from build123d import *

# Parameters (mm, degrees)
SKETCH1_W           = 120
SKETCH1_H           = 100
BOSS_EXTRUDE1_DEPTH = 20
SKETCH6_W           = 110
SKETCH6_H           = 40
CUT_EXTRUDE1_DEPTH  = 20
SKETCH6_3_W         = 5
SKETCH6_3_H         = 40
BOSS_EXTRUDE4_DEPTH = 20
SKETCH14_W          = 5
SKETCH14_H          = 5
CUT_EXTRUDE2_DEPTH  = 10
SKETCH15_W          = 10
SKETCH15_H          = 10
CUT_EXTRUDE3_DEPTH  = 10
SKETCH16_W          = 3
SKETCH16_H          = 3
SKETCH16_W_2        = 6
SKETCH16_H_2        = 6
CUT_EXTRUDE4_DEPTH  = 5


with BuildPart() as part:
    # Sketch1 → Boss-Extrude1 (new body)
    with BuildSketch(Plane(origin=(0, 0, 0), x_dir=(1, 0, 0), z_dir=(0, 1, 0))):
        Rectangle(SKETCH1_W, SKETCH1_H)
    extrude(amount=BOSS_EXTRUDE1_DEPTH)

    # Sketch6 → Cut-Extrude1 (cut)
    with BuildSketch(Plane.XZ):
        with Locations((0, 25)):
            Rectangle(SKETCH6_W, SKETCH6_H)
    extrude(amount=-CUT_EXTRUDE1_DEPTH, mode=Mode.SUBTRACT)

    # Sketch6_3 → Boss-Extrude4 (add)
    with BuildSketch(Plane.XZ):
        with Locations((-52.5, 25)):
            Rectangle(SKETCH6_3_W, SKETCH6_3_H)
        with Locations((52.5, 25)):
            Rectangle(SKETCH6_3_W, SKETCH6_3_H)
    extrude(amount=-BOSS_EXTRUDE4_DEPTH)

    # Sketch14 → Cut-Extrude2 (cut)
    with BuildSketch(Plane(origin=(0, 20, 0), x_dir=(1, 0, 0), z_dir=(0, 1, 0))):
        with Locations((-57.5, -7.820888862)):
            Rectangle(SKETCH14_W, SKETCH14_H)
        Polygon((-50, -0.320888862), (-60, -0.320888862), (-60, -5.320888862), (-55, -5.320888862), (-55, -10.320888862), (-50, -10.320888862), (-50, -5), align=None)
        Polygon((60, -5.320888862), (60, -0.320888862), (50, -0.320888862), (50, -5), (50, -10.320888862), (55, -10.320888862), (55, -5.320888862), align=None)
        with Locations((57.5, -7.820888862)):
            Rectangle(SKETCH14_W, SKETCH14_H)
    extrude(amount=-CUT_EXTRUDE2_DEPTH, mode=Mode.SUBTRACT)

    # Sketch15 → Cut-Extrude3 (cut)
    with BuildSketch(Plane(origin=(0, 20, 0), x_dir=(1, 0, 0), z_dir=(0, 1, 0))):
        with Locations((-55, 45)):
            Rectangle(SKETCH15_W, SKETCH15_H)
        with Locations((55, 45)):
            Rectangle(SKETCH15_W, SKETCH15_H)
        with Locations((55, -45)):
            Rectangle(SKETCH15_W, SKETCH15_H)
        with Locations((-55, -45)):
            Rectangle(SKETCH15_W, SKETCH15_H)
    extrude(amount=-CUT_EXTRUDE3_DEPTH, mode=Mode.SUBTRACT)

    # Sketch16 → Cut-Extrude4 (cut)
    with BuildSketch(Plane.XZ):
        with Locations((-57.5, 47.5)):
            Rectangle(SKETCH16_W, SKETCH16_H)
        with Locations((57.5, 47.5)):
            Rectangle(SKETCH16_W, SKETCH16_H)
        with Locations((-57.5, 2.5)):
            Rectangle(SKETCH16_W, SKETCH16_H)
        with Locations((57.5, 2.5)):
            Rectangle(SKETCH16_W, SKETCH16_H)
        with Locations((55, -25)):
            Rectangle(SKETCH16_W_2, SKETCH16_H_2)
        with Locations((-55, -25)):
            Rectangle(SKETCH16_W_2, SKETCH16_H_2)
    extrude(amount=-CUT_EXTRUDE4_DEPTH, mode=Mode.SUBTRACT)


solid = part.part
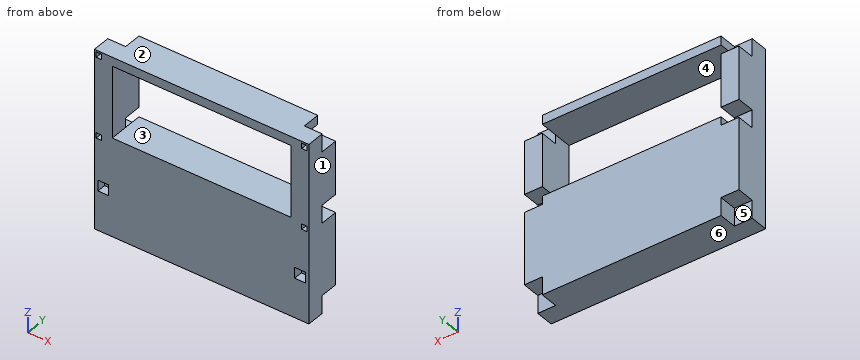
Geometry: final body of the model. Coordinates: model frame, mm. Face numbers are marked on the shaded views. A direction names the side the tool comes from. Round coordinates to 2 decimals unless told otherwise and drop trailing zeros. Write each loop counter-clockwise with the first axis right and the second up, starting at its lowest first coordinate (ties: lowest second). Pieces come first, ordered by that corner, then holes. Notation, with made-up numbers: M -6,63.25 L 44,63.25 A26 ccw 44,101.25 Z; hole C 85,-20 d5. An arc over 180 degrees is marked long. Write item = value, one per line.
Item 1: Section query C-C on y = 8.25. Return loops of the section in (x, z), then the cut area to 3 significant figures.
Findings:
outline = M -60,-50 L 60,-50 L 60,50 L -60,50 Z; hole M -50,5 L 50,5 L 50,45 L -50,45 Z
area = 8,000 mm^2
Item 2: Access query for the marked faces 4, 5 and 6. Directions: +Z, -Z, +X, -X, +Y, -Y. A direction counts if a zero-diameter tool reaches every point of the face in a straight line with its end or side. Return the directions, or none.
Findings:
face_4 = +Y, -Y
face_5 = -Z, -X, +Y
face_6 = -Z, +X, -X, +Y, -Y
Item 3: Section query A-A on x = 0.5. Return loops of the section in (y, z).
Findings:
outline = M 0,-50 L 20,-50 L 20,5 L 0,5 Z; M 0,45 L 20,45 L 20,50 L 0,50 Z
Item 4: Material intervals for line 1 along Z through (x, y) = (-12, 17.25); line 2 along Z through (x, y) = (50.5, 18); line 3 along X through (y, z) = (8, 15), sorted ascending. Write a range as [from, to].
Findings:
line_1 = [-50, 5], [45, 50]
line_2 = [-40, 0.32], [10.32, 40]
line_3 = [-60, -50], [50, 60]
Item 5: Pull-direction query (X, two-part tool) for the marked faces 1, 2 and 3; classes: pulls with the +X half, pulls with the -X half, needs draft (parallel to the pull), parting line crosses it, or undercut.
Findings:
face_1 = pulls with the +X half
face_2 = needs draft
face_3 = undercut
Item 6: Section query D-D on z = -26.5. Return loops of the section in (x, y).
Findings:
outline = M -60,0 L -58,0 L -58,5 L -52,5 L -52,0 L 52,0 L 52,5 L 58,5 L 58,0 L 60,0 L 60,20 L -60,20 Z
Item 7: Pin query (flat end, axial travel): P1, Ø3, axis at x = -55.5, z = -25, coming from the -Y side; P2, Ø5, axis at x = -56, y = 16, coming from the +Z side; P3, Ø5, axis at x = -57, y = 15, coming from the -Z side. Return the tip coordinate at first contact, or that it passes through.
Findings:
P1 = 5
P2 = 40
P3 = -40
Item 8: Section query B-B on z = 12. Return loops of the section in (x, y), then the cut area to 3 significant figures.
Findings:
outline = M -60,0 L -50,0 L -50,20 L -60,20 Z; M 50,0 L 60,0 L 60,20 L 50,20 Z
area = 400 mm^2
